Design review of the part built by this model. Coordinates are the model's own, in mm. Face numbers are marked on the shaded views. A direction names the side the tool comes from. Coordinates: 2 decimals unless noted, no trailing zeros. Loops run counter-clockwise (first coordinate to the right, second up) from the corner with the lowest first, then second, coordinate; pieces in that order, holes last.
Q1. Add section A-A on x = 16. Give the boundary of the cut face in (y, z), and give its area (3 significant figures).
Q2. Add section B-B on y = -2. Give the boundary of the cut face in (x, z), and give its area (3 significant figures).
Q3. Machinability: for the marked faces 3 and 4, which of the approach directions +Z, -Z, +X, -X, +Y, -Y give a long, thin tool a straight path to every point of the face, cutting with its end or side? Answer none if there is none.
Q4. Add section C-C on z = 15. Give the number of separate pieces and of enclosed holes in the cut face, and give its area (3 significant figures).
Q5. For P1, Ø6.5, axis at x = -9.54, y = -9.54, coming from the -Z side (3 decimals); P2, Ø2.5, axis at x = 8, y = -11, coming from the +Z side (3 decimals); P3, Ø1, axis at x = -8, z = 14, coming from the +Y side, all flat-tipped, find the tip position at first contact; note any pin that passes through.
Q6. Draft analysis for pull direction Y (two halves, no side actions). For the marked faces 1 and 2, state which applies: released by +Y, released by -Y, zero draft, split by the parting line, or undercut.
Q7. Wall thickness on probe 1 along X at (y, z) = (-0.5, 11.5); probe 2 along Y at (x, z) = (-6, 16): over which ranges is each line inside the solid? List them lowest first.
```python
from build123d import *

# Parameters (mm, degrees)
F0_R      = 19.05
F0_R_2    = 2.15265
F1_DEPTH  = 66.04
F4_R      = 3.96875
F5_DEPTH  = 62.865
F6_R      = 3.96875
F7_DEPTH  = 61.595
F9_DEPTH  = 66.04
F10_COUNT = 4
F10_ANGLE = 270


with BuildPart() as f1:
    # F0 (on Top) → F1 (new body)
    with BuildSketch(Plane.XY):
        Circle(F0_R)
        with Locations((-9.5415221286, -9.5415221286)):
            Circle(F0_R_2, mode=Mode.SUBTRACT)
        with Locations((9.5415221286, -9.5415221286)):
            Circle(F0_R_2, mode=Mode.SUBTRACT)
        with Locations((-9.5415221286, 9.5415221286)):
            Circle(F0_R_2, mode=Mode.SUBTRACT)
        with BuildLine():
            ThreePointArc((0, 7.9375), (5.6126600757, 5.6126600757), (7.9375, 0))
            ThreePointArc((7.9375, 0), (-5.6126600757, -5.6126600757), (0, 7.9375))
        make_face(mode=Mode.SUBTRACT)
        with Locations((9.5415221286, 9.5415221286)):
            Circle(F0_R_2, mode=Mode.SUBTRACT)
    extrude(amount=F1_DEPTH)

    # F4 (on face) → F5 (cut, through all)
    with BuildSketch(Plane(origin=(0, 0, 0), x_dir=(1, 0, 0), z_dir=(0, 0, -1))):
        with Locations((9.5415221286, -9.5415221286)):
            Circle(F4_R)
        with Locations((-9.5415221286, 9.5415221286)):
            Circle(F4_R)
    extrude(amount=-F5_DEPTH, mode=Mode.SUBTRACT)

    # F6 (on face) → F7 (cut, through all)
    with BuildSketch(Plane.XY.offset(66.04)):
        with Locations((-9.5415221286, 9.5415221286)):
            Circle(F6_R)
        with Locations((9.5415221286, -9.5415221286)):
            Circle(F6_R)
    extrude(amount=-F7_DEPTH, mode=Mode.SUBTRACT)

    # F8 (on face) → F9 (cut, through all)
    with BuildSketch(Plane(origin=(0, 0, 0), x_dir=(1, 0, 0), z_dir=(0, 0, -1))):
        with BuildLine():
            ThreePointArc((8.8488960712, -15.0544327217), (5.6543471209, -13.5116335278), (4.0444600337, -10.350362278))
            ThreePointArc((4.0444600337, -10.350362278), (0, -11.1125), (-4.0444600337, -10.350362278))
            ThreePointArc((-4.0444600337, -10.350362278), (-5.6543471209, -13.5116335278), (-8.8488960712, -15.0544327217))
            ThreePointArc((-8.8488960712, -15.0544327217), (0, -17.4625), (8.8488960712, -15.0544327217))
        make_face()
    f9 = extrude(amount=-F9_DEPTH, mode=Mode.SUBTRACT)

    # F10: F9 ×4 about axis
    f10_axis = Axis((0, 0, 0), (0, 0, -1))
    for i in range(1, F10_COUNT):
        add(f9.rotate(f10_axis, i * F10_ANGLE / (F10_COUNT - 1)), mode=Mode.SUBTRACT)


solid = f1.part
```
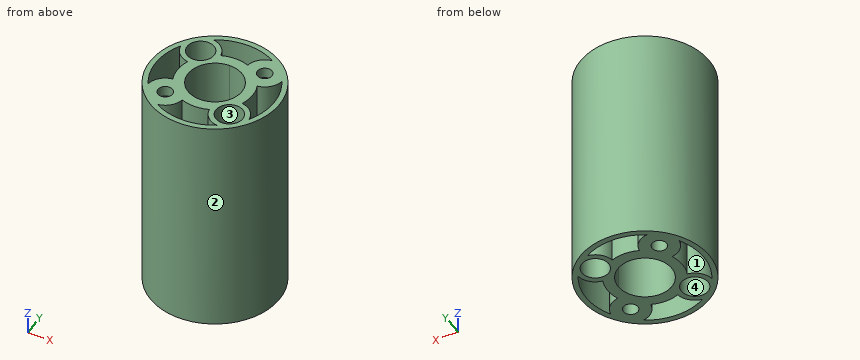
Entries:
1. outline: (-10.34, 0) - (-7, 0) - (-7, 66.04) - (-10.34, 66.04) - close; (7, 0) - (10.34, 0) - (10.34, 66.04) - (7, 66.04) - close
1. area: 442 mm2
2. outline: (-18.94, 0) - (-17.35, 0) - (-17.35, 66.04) - (-18.94, 66.04) - close; (-10.93, 0) - (-7.68, 0) - (-7.68, 66.04) - (-10.93, 66.04) - close; (7.68, 0) - (10.93, 0) - (10.93, 66.04) - (7.68, 66.04) - close; (17.35, 0) - (18.94, 0) - (18.94, 66.04) - (17.35, 66.04) - close
2. area: 640 mm2
3. face 3: +Z
3. face 4: -Z
4. separate pieces: 1
4. enclosed holes: 9
4. area: 444 mm2
5. P1: stops at z = 62.865
5. P2: stops at z = 4.445
5. P3: stops at y = 17.51
6. face 1: undercut
6. face 2: split by the parting line
7. probe 1: x = -19.04 to -17.46, -11.1 to -7.92, 7.92 to 11.1, 17.46 to 19.04
7. probe 2: y = -18.08 to -16.4, -13.82 to -11.33, -7.75 to -5.2, 5.2 to 7.75, 11.33 to 13.82, 16.4 to 18.08
